from build123d import *

# Parameters (mm, degrees)
SKETCH1_R           = 1.925
BOSS_EXTRUDE1_DEPTH = 4
FILLET1_R           = 3


with BuildPart() as part:
    # Sketch1 → Boss-Extrude1 (new body)
    with BuildSketch(Plane.XY):
        with BuildLine():
            Line((-7.5, 7.5), (7.5, 7.5))
            ThreePointArc((7.5, 7.5), (15, 0), (7.5, -7.5))
            Line((7.5, -7.5), (-7.5, -7.5))
            ThreePointArc((-7.5, -7.5), (-15, 0), (-7.5, 7.5))
        make_face()
        with Locations((7.5, 0)):
            Circle(SKETCH1_R, mode=Mode.SUBTRACT)
        with Locations((-7.5, 0)):
            Circle(SKETCH1_R, mode=Mode.SUBTRACT)
    extrude(amount=BOSS_EXTRUDE1_DEPTH)

    # Sketch3 → Revolve1 (revolve)
    with BuildSketch(Plane(origin=(0, 0, 0), x_dir=(1, 0, 0), z_dir=(0, 1, 0))):
        with BuildLine():
            Line((0, 11.25), (0, 7.5))
            Line((0, 7.5), (1.75, 7.5))
            Line((1.75, 7.5), (2.063144305, 4.36855695))
            ThreePointArc((2.063144305, 4.36855695), (3.592033647, 8.576937454), (0, 11.25))
        make_face()
        with BuildLine():
            Line((1.75, 7.5), (0, 7.5))
            Line((0, 7.5), (0, 3.75))
            ThreePointArc((0, 3.75), (1.076937454, 3.907966353), (2.063144305, 4.36855695))
            Line((2.063144305, 4.36855695), (1.75, 7.5))
        make_face()
        with BuildLine():
            ThreePointArc((2.063144305, 4.36855695), (1.076937454, 3.907966353), (0, 3.75))
            Line((0, 3.75), (0, 0))
            Line((0, 0), (2.5, 0))
            Line((2.5, 0), (2.063144305, 4.36855695))
        make_face()
    revolve(axis=Axis((0, 0, 0), (0, 0, -1)))

    # Fillet1
    fillet1_edges = [part.edges().sort_by_distance(p)[0] for p in [
        (-2.5, 0, 0),
    ]]
    fillet(fillet1_edges, radius=FILLET1_R)


solid = part.part
The listing builds one solid part. Answer for the finished solid, in the listing's coordinates (mm). A direction names the side the tool comes from. Give positions to 0.01 mm unless a question says otherwise; leave off trailing zeros. Write each loop counter-clockwise with the first axis right and the second up, starting at its lowest first coordinate (ties: lowest second). Pieces come first, ordered by that corner, then holes. Notation, with made-up numbers: (-6.75, 62.5) -> (8.25, 62.5) arc R27 cw to (8.25, 99.5) -> close; hole circle Ø3 at (-38.5, -7). An arc over 180 degrees is marked (long way). One line per question, with ' | ' between items. Start each with the question number.
1. Section C-C (z = -4) is taken. Determine the outline of the cut face in (x, y), plus the area to 3 significant figures.
2. For a pull along X with two mould halves and no side action, classify faces 3 (the flat face through (0, -7.5, 2)), 4 (the cylindrical face through (5.577, 0.085, 1.972)), 5 (the cylindrical face through (15, 0, 2)) as pulls with the +X half, pulls with the -X half, needs draft (parallel to the pull), parting line crosses it, or undercut.
3. Section A-A (y = 0) is taken. Determine the outline of the cut face in (x, z) (3 decimals), plus the area to 3 significant figures.
4. Section B-B (z = 2) is taken. Determine the outline of the cut face in (x, y) (3 decimals), plus the area to 3 significant figures.
5. For faces 1 (the flat face through (0, 0, 4)), 2 (the conical face through (-0.28, -2.11, -3.73)), determine the directions among +Z, -Z, +X, -X, +Y, -Y from which every point of the face is accessible in a straight line to the end or side of a thin tool.
6. Given pin 1 Ø8 at (y, z) = (-1, -6) entering from +X; pin 2 Ø1 at (x, y) = (7, -4.5) entering from -Z; pin 3 Ø5 at (y, z) = (-2.5, -7.5) entering from -X, each flat-ended and moving along its own axis, determine where each tip first touches the part or whether it passes through.
7. Section D-D (x = 0) is taken. Determine the outline of the cut face in (y, z), plus the area to 3 significant figures.
8. Find the intervals of material crossed by probe 1 along Y at (x, z) = (7.5, 1.1) (3 decimals); probe 2 along X at (y, z) = (-1.25, 1.5); probe 3 along Z at (x, y) = (13.5, -0.75), in increasing order.
Response values:
1) outline: circle Ø4.2 at (0, 0) | area: 13.9 mm2
2) face 3: needs draft | face 4: undercut | face 5: pulls with the +X half
3) outline: (-15, 0) -> (-9.425, 0) -> (-9.425, 4) -> (-15, 4) -> close; (-5.575, 0) -> (-5.215, 0) arc R3 cw to (-2.23, -2.701) -> (-2.063, -4.369) arc R3.75 ccw (long way) to (2.063, -4.369) -> (2.23, -2.701) arc R3 cw to (5.215, 0) -> (5.575, 0) -> (5.575, 4) -> (-5.575, 4) -> close; (9.425, 0) -> (15, 0) -> (15, 4) -> (9.425, 4) -> close | area: 155 mm2
4) outline: (-7.5, -7.5) -> (7.5, -7.5) arc R7.5 ccw to (7.5, 7.5) -> (-7.5, 7.5) arc R7.5 ccw to start; hole circle Ø3.85 at (-7.5, 0); hole circle Ø3.85 at (7.5, 0) | area: 378 mm2
5) face 1: +Z, +X, -X, +Y, -Y | face 2: none
6) pin 1: x = 3.75 | pin 2: z = 0 | pin 3: x = -3.75
7) outline: (-7.5, 0) -> (-5.21, 0) arc R3 cw to (-2.23, -2.7) -> (-2.06, -4.37) arc R3.75 ccw (long way) to (2.06, -4.37) -> (2.23, -2.7) arc R3 cw to (5.21, 0) -> (7.5, 0) -> (7.5, 4) -> (-7.5, 4) -> close | area: 125 mm2
8) probe 1: -7.5 to -1.925, 1.925 to 7.5 | probe 2: -14.9 to -8.96, -6.04 to 6.04, 8.96 to 14.9 | probe 3: 0 to 4
